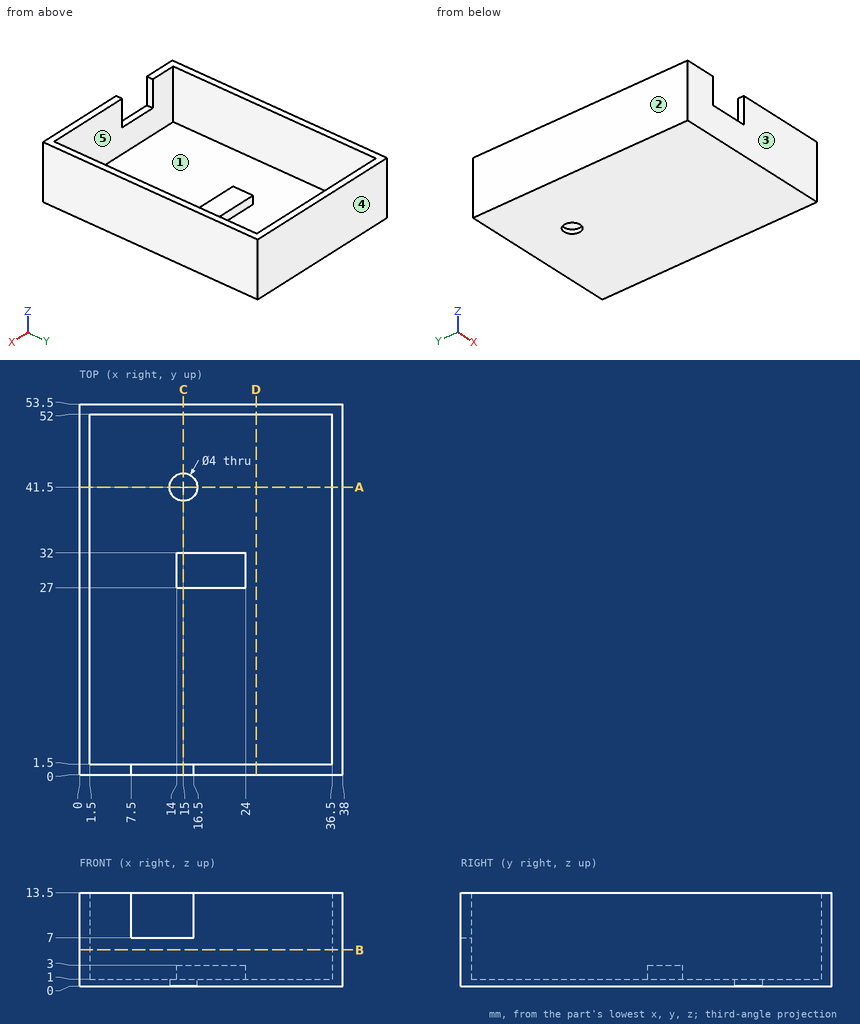
Verification items for this drawing (mm, ordinates from the low corner). A direction names the side the tool comes from. Round coordinates to 2 decimals unless told otherwise and drop trailing zeros. Write each loop counter-clockwise with the first axis right and the second up, starting at its lowest first coordinate (ties: lowest second). Pieces come first, ordered by that corner, then holes. Notation, with made-up numbers: (-29, 30.25) - (28, 30.25) arc R16 cw to (28, 44.25) - close; hole circle Ø3 at (21, -10.5). An arc over 180 degrees is marked (long way). Answer as a JSON object with one key per item and string values. Group by question number.
Q1. Section check B-B, the plane z = 5.25. Enter the section's corners in (x, y).
Q2. Section check C-C, the plane x = 15. Enter the section's corners in (y, z), plus the area to 4 significant figures.
Q3. Go/stop test with flat-tipped pins: pin 1 Ø8 at (x, y) = (18, 11.5) entering from +Z; pin 2 Ø5 at (x, z) = (17.5, 7) entering from -Y; pin 3 Ø10.5 at (x, y) = (16.5, 33.5) entering from +Z; pin 4 Ø0.8 at (x, y) = (11, 1) entering from +Z. Record where each tip stops, or that it passes through.
Q4. Mould release check, pull along X, two halves, no side actions. Record for the marked faces 1, 2 and 3: released by +X, released by -X, zero draft, split by the parting line, or undercut.
Q5. Section check D-D, the plane x = 25.5. Enter the section's corners in (y, z), plus the area to 3 significant figures.
Q6. Section check A-A, the plane y = 41.5. Enter the section's corners in (x, z).
Q7. Thickness scan on line 1 (Y direction, x = 18, z = 2.75); line 2 (Y direction, x = 15, z = 0.4); line 3 (Y direction, x = 5, z = 4). Record the ranges inside material, lowest first.
Q8. Tool access check on the marked faces 4 and 5. Record the directions out of +Z, -Z, +X, -X, +Y, -Y that give a thin tool (end or side, any length) a straight path to the whole face; none if there is none.
Found:
{
 "1": {"outline": "(0, 0) - (38, 0) - (38, 53.5) - (0, 53.5) - close; hole (1.5, 1.5) - (36.5, 1.5) - (36.5, 52) - (1.5, 52) - close"},
 "2": {"outline": "(0, 0) - (39.5, 0) - (39.5, 1) - (32, 1) - (32, 3) - (27, 3) - (27, 1) - (1.5, 1) - (1.5, 7) - (0, 7) - close; (43.5, 0) - (53.5, 0) - (53.5, 13.5) - (52, 13.5) - (52, 1) - (43.5, 1) - close", "area": "87.25 mm^2"},
 "3": {"pin 1": "stops at z = 1", "pin 2": "stops at y = 0", "pin 3": "stops at z = 3", "pin 4": "stops at z = 7"},
 "4": {"face 1": "undercut", "face 2": "released by -X", "face 3": "zero draft"},
 "5": {"outline": "(0, 0) - (53.5, 0) - (53.5, 13.5) - (52, 13.5) - (52, 1) - (1.5, 1) - (1.5, 13.5) - (0, 13.5) - close", "area": "91.0 mm^2"},
 "6": {"outline": "(0, 0) - (13, 0) - (13, 1) - (1.5, 1) - (1.5, 13.5) - (0, 13.5) - close; (17, 0) - (38, 0) - (38, 13.5) - (36.5, 13.5) - (36.5, 1) - (17, 1) - close"},
 "7": {"line 1": "y = 0 to 1.5, 27 to 32, 52 to 53.5", "line 2": "y = 0 to 39.5, 43.5 to 53.5", "line 3": "y = 0 to 1.5, 52 to 53.5"},
 "8": {"face 4": "+Z, -Z, +X, -X, +Y", "face 5": "+Z"}
}
